Geometry check sheet. Reference: the model listing, model coordinates, mm. A direction names the side the tool comes from. Give positions to 0.01 mm unless a question says otherwise; leave off trailing zeros. Loops run counter-clockwise (first coordinate to the right, second up) from the corner with the lowest first, then second, coordinate; pieces in that order, holes last. Notation, with made-up numbers: (36.25, 70.25) - (95.25, 70.25) arc R19 cw to (95.25, 78.25) - close; hole circle Ø8 at (44, 68.25). An arc over 180 degrees is marked (long way). One line per question, with ' | ' between items. Start each with the question number.
from build123d import *

# Parameters (mm, degrees)
SKETCH1_R           = 1.25
SKETCH1_R_2         = 0.75
SKETCH1_W           = 60
SKETCH1_H           = 20
SKETCH1_W_2         = 5
SKETCH1_H_2         = 1
BOSS_EXTRUDE2_DEPTH = 3
SKETCH4_R           = 0.75
CUT_EXTRUDE3_DEPTH  = 3
SKETCH5_R           = 0.75
CUT_EXTRUDE4_DEPTH  = 3
SKETCH14_R          = 0.75
CUT_EXTRUDE12_DEPTH = 10
BOSS_EXTRUDE4_START = -3
SKETCH15_R          = 0.75
BOSS_EXTRUDE4_DEPTH = 3
SKETCH20_R          = 1.25
CUT_EXTRUDE17_DEPTH = 3
SKETCH23_R          = 0.75
CUT_EXTRUDE21_DEPTH = 10
SKETCH25_W          = 10
SKETCH25_H          = 1
CUT_EXTRUDE23_DEPTH = 3
SKETCH26_R          = 1.25
CUT_EXTRUDE24_DEPTH = 3
SKETCH29_R          = 1.25
CUT_EXTRUDE27_DEPTH = 3
SKETCH33_W          = 5
SKETCH33_H          = 2
CUT_EXTRUDE31_DEPTH = 3
SKETCH34_W          = 5
SKETCH34_H          = 2
CUT_EXTRUDE32_DEPTH = 3
SKETCH35_R          = 1.25
CUT_EXTRUDE33_DEPTH = 3
SKETCH37_R          = 1.25
CUT_EXTRUDE34_DEPTH = 3
SKETCH38_R          = 1.25
CUT_EXTRUDE35_DEPTH = 3
SKETCH41_R          = 0.75
CUT_EXTRUDE38_DEPTH = 3
SKETCH42_W          = 6
SKETCH42_H          = 2
CUT_EXTRUDE40_DEPTH = 3
SKETCH43_W          = 6
SKETCH43_H          = 2
CUT_EXTRUDE41_DEPTH = 3
BOSS_EXTRUDE5_START = -3
SKETCH45_R          = 1.25
BOSS_EXTRUDE5_DEPTH = 3
BOSS_EXTRUDE6_START = -3
SKETCH46_R          = 1.25
BOSS_EXTRUDE6_DEPTH = 3
SKETCH47_R          = 1.25
CUT_EXTRUDE42_DEPTH = 3
SKETCH49_R          = 1.25
CUT_EXTRUDE43_DEPTH = 3
SKETCH51_R          = 1.25
CUT_EXTRUDE44_DEPTH = 3
SKETCH52_R          = 1.25
CUT_EXTRUDE45_DEPTH = 3
SKETCH53_R          = 1.25
CUT_EXTRUDE46_DEPTH = 3
SKETCH54_R          = 1.25
CUT_EXTRUDE47_DEPTH = 3
SKETCH55_W          = 20
SKETCH55_H          = 1
CUT_EXTRUDE48_DEPTH = 10
SKETCH56_R          = 0.75
CUT_EXTRUDE49_DEPTH = 10
SKETCH57_R          = 0.75
CUT_EXTRUDE50_DEPTH = 10
SKETCH59_R          = 1.5
CUT_EXTRUDE51_DEPTH = 10
SKETCH60_R          = 0.75
CUT_EXTRUDE52_DEPTH = 10
SKETCH61_R          = 0.75
CUT_EXTRUDE53_DEPTH = 10
SKETCH65_R          = 1.5
CUT_EXTRUDE55_DEPTH = 10
SKETCH66_R          = 1.5
CUT_EXTRUDE56_DEPTH = 10
SKETCH67_R          = 1.5
CUT_EXTRUDE57_DEPTH = 10
CUT_EXTRUDE58_DEPTH = 10
CUT_EXTRUDE59_DEPTH = 10
BOSS_EXTRUDE7_DEPTH = 3


with BuildPart() as part:
    # Sketch1 → Boss-Extrude2 (new body)
    with BuildSketch(Plane.XY):
        Polygon((58.345821786, 13.119852123), (58.345821786, -56.880147877), (-191.654178214, -56.880147877), (-191.654178214, -26.880147877), (-221.654178214, -6.880147877), (-221.654178214, 33.119852123), (-121.654178214, 33.119852123), (-91.654178214, 13.119852123), align=None)
        with Locations((53.345821786, 7.945541925)):
            Circle(SKETCH1_R, mode=Mode.SUBTRACT)
        with Locations((53.345821786, -52.054458075)):
            Circle(SKETCH1_R, mode=Mode.SUBTRACT)
        with Locations((25.505821786, -18.330147877)):
            Circle(SKETCH1_R_2, mode=Mode.SUBTRACT)
        with Locations((-181.654178214, 13.119852123)):
            Rectangle(SKETCH1_W, SKETCH1_H, mode=Mode.SUBTRACT)
        with Locations((25.845821786, 10.619852123)):
            Rectangle(SKETCH1_W_2, SKETCH1_H_2, mode=Mode.SUBTRACT)
        with Locations((40.845821786, 10.619852123)):
            Rectangle(SKETCH1_W_2, SKETCH1_H_2, mode=Mode.SUBTRACT)
    extrude(amount=BOSS_EXTRUDE2_DEPTH)

    # Sketch4 → Cut-Extrude3 (cut)
    with BuildSketch(Plane.XY.offset(3)):
        with Locations((-12.554178214, -8.780147877)):
            Circle(SKETCH4_R)
    extrude(amount=-CUT_EXTRUDE3_DEPTH, mode=Mode.SUBTRACT)

    # Sketch5 → Cut-Extrude4 (cut)
    with BuildSketch(Plane.XY.offset(3)):
        with Locations((-13.994178214, -15.020147877)):
            Circle(SKETCH5_R)
    extrude(amount=-CUT_EXTRUDE4_DEPTH, mode=Mode.SUBTRACT)

    # Sketch14 → Cut-Extrude12 (cut)
    with BuildSketch(Plane.XY.offset(3)):
        with Locations((25.505821786, -20.330147877)):
            Circle(SKETCH14_R)
        with Locations((25.505821786, -26.730147877)):
            Circle(SKETCH14_R)
    extrude(amount=-CUT_EXTRUDE12_DEPTH, mode=Mode.SUBTRACT)

    # Sketch15 → Boss-Extrude4 (add)
    with BuildSketch(Plane.XY.offset(3).offset(BOSS_EXTRUDE4_START)):
        with Locations((25.505821786, -18.330147877)):
            Circle(SKETCH15_R)
    extrude(amount=BOSS_EXTRUDE4_DEPTH)

    # Sketch20 → Cut-Extrude17 (cut)
    with BuildSketch(Plane.XY.offset(3)):
        with Locations((-16.654178214, 4.119852123)):
            Circle(SKETCH20_R)
    extrude(amount=-CUT_EXTRUDE17_DEPTH, mode=Mode.SUBTRACT)

    # Sketch23 → Cut-Extrude21 (cut)
    with BuildSketch(Plane.XY.offset(3)):
        with Locations((-93.524701832, -7.521447448)):
            Circle(SKETCH23_R)
    extrude(amount=-CUT_EXTRUDE21_DEPTH, mode=Mode.SUBTRACT)

    # Sketch25 → Cut-Extrude23 (cut)
    with BuildSketch(Plane.XY.offset(3)):
        with Locations((33.345821786, 10.619852123)):
            Rectangle(SKETCH25_W, SKETCH25_H)
    extrude(amount=-CUT_EXTRUDE23_DEPTH, mode=Mode.SUBTRACT)

    # Sketch26 → Cut-Extrude24 (cut)
    with BuildSketch(Plane.XY.offset(3)):
        with Locations((-97.444178214, 7.419852123)):
            Circle(SKETCH26_R)
    extrude(amount=-CUT_EXTRUDE24_DEPTH, mode=Mode.SUBTRACT)

    # Sketch29 → Cut-Extrude27 (cut)
    with BuildSketch(Plane.XY.offset(3)):
        with Locations((-176.654178214, -41.880147877)):
            Circle(SKETCH29_R)
    extrude(amount=-CUT_EXTRUDE27_DEPTH, mode=Mode.SUBTRACT)

    # Sketch33 → Cut-Extrude31 (cut)
    with BuildSketch(Plane.XY.offset(3)):
        with Locations((-129.154178214, 30.119852123)):
            Rectangle(SKETCH33_W, SKETCH33_H)
    extrude(amount=-CUT_EXTRUDE31_DEPTH, mode=Mode.SUBTRACT)

    # Sketch34 → Cut-Extrude32 (cut)
    with BuildSketch(Plane.XY.offset(3)):
        with Locations((-144.154178214, 30.119852123)):
            Rectangle(SKETCH34_W, SKETCH34_H)
    extrude(amount=-CUT_EXTRUDE32_DEPTH, mode=Mode.SUBTRACT)

    # Sketch35 → Cut-Extrude33 (cut)
    with BuildSketch(Plane.XY.offset(3)):
        with Locations((-123.654178214, 30.119852123)):
            Circle(SKETCH35_R)
        with Locations((-149.654178214, 30.119852123)):
            Circle(SKETCH35_R)
    extrude(amount=-CUT_EXTRUDE33_DEPTH, mode=Mode.SUBTRACT)

    # Sketch37 → Cut-Extrude34 (cut)
    with BuildSketch(Plane.XY.offset(3)):
        with Locations((-61.654178214, -1.880147877)):
            Circle(SKETCH37_R)
    extrude(amount=-CUT_EXTRUDE34_DEPTH, mode=Mode.SUBTRACT)

    # Sketch38 → Cut-Extrude35 (cut)
    with BuildSketch(Plane.XY.offset(3)):
        with Locations((-87.444178214, -25.580147877)):
            Circle(SKETCH38_R)
    extrude(amount=-CUT_EXTRUDE35_DEPTH, mode=Mode.SUBTRACT)

    # Sketch41 → Cut-Extrude38 (cut)
    with BuildSketch(Plane.XY.offset(3)):
        with Locations((-112.306137726, -10.395062897)):
            Circle(SKETCH41_R)
    extrude(amount=-CUT_EXTRUDE38_DEPTH, mode=Mode.SUBTRACT)

    # Sketch42 → Cut-Extrude40 (cut)
    with BuildSketch(Plane.XY.offset(3)):
        with Locations((-105.524701832, -12.521447448)):
            Rectangle(SKETCH42_W, SKETCH42_H)
    extrude(amount=-CUT_EXTRUDE40_DEPTH, mode=Mode.SUBTRACT)

    # Sketch43 → Cut-Extrude41 (cut)
    with BuildSketch(Plane.XY.offset(3)):
        with Locations((-105.524701832, 14.478552552)):
            Rectangle(SKETCH43_W, SKETCH43_H)
    extrude(amount=-CUT_EXTRUDE41_DEPTH, mode=Mode.SUBTRACT)

    # Sketch45 → Boss-Extrude5 (add)
    with BuildSketch(Plane.XY.offset(3).offset(BOSS_EXTRUDE5_START)):
        with Locations((53.345821786, -52.054458075)):
            Circle(SKETCH45_R)
    extrude(amount=BOSS_EXTRUDE5_DEPTH)

    # Sketch46 → Boss-Extrude6 (add)
    with BuildSketch(Plane.XY.offset(3).offset(BOSS_EXTRUDE6_START)):
        with Locations((53.345821786, 7.945541925)):
            Circle(SKETCH46_R)
    extrude(amount=BOSS_EXTRUDE6_DEPTH)

    # Sketch47 → Cut-Extrude42 (cut)
    with BuildSketch(Plane.XY.offset(3)):
        with Locations((53.345821786, 8.119852123)):
            Circle(SKETCH47_R)
    extrude(amount=-CUT_EXTRUDE42_DEPTH, mode=Mode.SUBTRACT)

    # Sketch49 → Cut-Extrude43 (cut)
    with BuildSketch(Plane.XY.offset(3)):
        with Locations((53.345821786, -10.880147877)):
            Circle(SKETCH49_R)
    extrude(amount=-CUT_EXTRUDE43_DEPTH, mode=Mode.SUBTRACT)

    # Sketch51 → Cut-Extrude44 (cut)
    with BuildSketch(Plane.XY.offset(3)):
        with Locations((53.345821786, -36.880147877)):
            Circle(SKETCH51_R)
    extrude(amount=-CUT_EXTRUDE44_DEPTH, mode=Mode.SUBTRACT)

    # Sketch52 → Cut-Extrude45 (cut)
    with BuildSketch(Plane.XY.offset(3)):
        with Locations((53.345821786, -51.880147877)):
            Circle(SKETCH52_R)
    extrude(amount=-CUT_EXTRUDE45_DEPTH, mode=Mode.SUBTRACT)

    # Sketch53 → Cut-Extrude46 (cut)
    with BuildSketch(Plane.XY.offset(3)):
        with Locations((-6.654178214, -51.880147877)):
            Circle(SKETCH53_R)
    extrude(amount=-CUT_EXTRUDE46_DEPTH, mode=Mode.SUBTRACT)

    # Sketch54 → Cut-Extrude47 (cut)
    with BuildSketch(Plane.XY.offset(3)):
        with Locations((-61.654178214, -51.880147877)):
            Circle(SKETCH54_R)
    extrude(amount=-CUT_EXTRUDE47_DEPTH, mode=Mode.SUBTRACT)

    # Sketch55 → Cut-Extrude48 (cut)
    with BuildSketch(Plane.XY.offset(3)):
        with Locations((33.345821786, 9.619852123)):
            Rectangle(SKETCH55_W, SKETCH55_H)
    extrude(amount=-CUT_EXTRUDE48_DEPTH, mode=Mode.SUBTRACT)

    # Sketch56 → Cut-Extrude49 (cut)
    with BuildSketch(Plane.XY.offset(3)):
        with Locations((-61.804178214, -20.030147877)):
            Circle(SKETCH56_R)
    extrude(amount=-CUT_EXTRUDE49_DEPTH, mode=Mode.SUBTRACT)

    # Sketch57 → Cut-Extrude50 (cut)
    with BuildSketch(Plane.XY.offset(3)):
        with Locations((-79.304178214, -20.030147877)):
            Circle(SKETCH57_R)
    extrude(amount=-CUT_EXTRUDE50_DEPTH, mode=Mode.SUBTRACT)

    # Sketch59 → Cut-Extrude51 (cut)
    with BuildSketch(Plane.XY.offset(3)):
        with Locations((-87.444178214, -42.580147877)):
            Circle(SKETCH59_R)
    extrude(amount=-CUT_EXTRUDE51_DEPTH, mode=Mode.SUBTRACT)

    # Sketch60 → Cut-Extrude52 (cut)
    with BuildSketch(Plane.XY.offset(3)):
        with Locations((-18.804178214, -26.030147877)):
            Circle(SKETCH60_R)
    extrude(amount=-CUT_EXTRUDE52_DEPTH, mode=Mode.SUBTRACT)

    # Sketch61 → Cut-Extrude53 (cut)
    with BuildSketch(Plane.XY.offset(3)):
        with Locations((-36.304178214, -26.030147877)):
            Circle(SKETCH61_R)
    extrude(amount=-CUT_EXTRUDE53_DEPTH, mode=Mode.SUBTRACT)

    # Sketch65 → Cut-Extrude55 (cut)
    with BuildSketch(Plane.XY.offset(3)):
        with Locations((1.345821786, 3.119852123)):
            Circle(SKETCH65_R)
    extrude(amount=-CUT_EXTRUDE55_DEPTH, mode=Mode.SUBTRACT)

    # Sketch66 → Cut-Extrude56 (cut)
    with BuildSketch(Plane.XY.offset(3)):
        with Locations((-107.444178214, -29.580147877)):
            Circle(SKETCH66_R)
    extrude(amount=-CUT_EXTRUDE56_DEPTH, mode=Mode.SUBTRACT)

    # Sketch67 → Cut-Extrude57 (cut)
    with BuildSketch(Plane.XY.offset(3)):
        with Locations((-127.444178214, -20.580147877)):
            Circle(SKETCH67_R)
    extrude(amount=-CUT_EXTRUDE57_DEPTH, mode=Mode.SUBTRACT)

    # Sketch68 → Cut-Extrude58 (cut)
    with BuildSketch(Plane.XY.offset(3)):
        with BuildLine():
            Line((-221.654178214, 33.119852123), (-216.654178214, 33.119852123))
            ThreePointArc((-216.654178214, 33.119852123), (-220.18971212, 31.655386029), (-221.654178214, 28.119852123))
            Line((-221.654178214, 28.119852123), (-221.654178214, 33.119852123))
        make_face()
    extrude(amount=-CUT_EXTRUDE58_DEPTH, mode=Mode.SUBTRACT)

    # Sketch69 → Cut-Extrude59 (cut)
    with BuildSketch(Plane.XY.offset(3)):
        with BuildLine():
            Line((-191.654178214, -56.880147877), (-191.654178214, -51.880147877))
            ThreePointArc((-191.654178214, -51.880147877), (-190.18971212, -55.415681783), (-186.654178214, -56.880147877))
            Line((-186.654178214, -56.880147877), (-191.654178214, -56.880147877))
        make_face()
    extrude(amount=-CUT_EXTRUDE59_DEPTH, mode=Mode.SUBTRACT)

    # Sketch72 → Boss-Extrude7 (add)
    with BuildSketch(Plane.XY.offset(3)):
        with BuildLine():
            Line((-211.654178214, 23.119852123), (-211.654178214, 18.119852123))
            ThreePointArc((-211.654178214, 18.119852123), (-210.18971212, 21.655386029), (-206.654178214, 23.119852123))
            Line((-206.654178214, 23.119852123), (-211.654178214, 23.119852123))
        make_face()
        with BuildLine():
            Line((-211.654178214, 3.119852123), (-211.654178214, 8.119852123))
            ThreePointArc((-211.654178214, 8.119852123), (-210.18971212, 4.584318217), (-206.654178214, 3.119852123))
            Line((-206.654178214, 3.119852123), (-211.654178214, 3.119852123))
        make_face()
        with BuildLine():
            Line((-151.654178214, 23.119852123), (-156.654178214, 23.119852123))
            ThreePointArc((-156.654178214, 23.119852123), (-153.118644308, 21.655386029), (-151.654178214, 18.119852123))
            Line((-151.654178214, 18.119852123), (-151.654178214, 23.119852123))
        make_face()
        with BuildLine():
            Line((-151.654178214, 3.119852123), (-156.654178214, 3.119852123))
            ThreePointArc((-156.654178214, 3.119852123), (-153.118644308, 4.584318217), (-151.654178214, 8.119852123))
            Line((-151.654178214, 8.119852123), (-151.654178214, 3.119852123))
        make_face()
    extrude(amount=-BOSS_EXTRUDE7_DEPTH)


solid = part.part
(1) Section check C-C, the plane z = 1.7. Count the separate pieces of the cut face and the enclosed holes in it, and give its area (3 significant figures).
(2) Material ranges on line 1 (Y direction, x = -174.5, z = 2.4); line 2 (X direction, y = 8, z = 2.4); line 3 (X direction, y = 29, z = 2.05), recorded low to high.
(3) Section check B-B, the plane x = -204. Record the boundary of the cut face in (y, z).
(4) Tool access check on faces 5 (the face through (-210.228, 4.623, 1.521)), 6 (the face through (-190.228, -55.377, 1.521)). Record the directions out of +Z, -Z, +X, -X, +Y, -Y that give a thin tool (end or side, any length) a straight path to the whole face; none if there is none.
(5) Section check A-A, the plane x = 30. Record the boundary of the cut face in (y, z).
(6) Mould release check, pull along X, two halves, no side actions. Record for faces 1 (the face through (-206.444, -17.02, 1.479)), 2 (the face through (-153.158, 21.694, 1.521)), 3 (the face through (-84, -21, 3)), 4 (the face through (-153.158, 4.546, 1.521)): pulls with the +X half, pulls with the -X half, needs draft (parallel to the pull), parting line crosses it, or undercut.
(7) Depth check by flat-ended pin: pin 1 Ø1.5 at (x, z) = (-104.5, 1) entering from +Y. Enter the tip coordinate at first touch or a pass-through.
Numbers:
1) separate pieces: 1 | enclosed holes: 33 | area: 19,300 mm^2
2) line 1: -56.88 to 3.12, 23.12 to 33.12 | line 2: -221.65 to -211.65, -151.66 to -98.55, -96.34 to 52.1, 54.59 to 58.35 | line 3: -221.58 to -150.21, -149.1 to -124.21, -123.1 to -115.47
3) outline: (-18.65, 0) - (3.12, 0) - (3.12, 3) - (-18.65, 3) - close; (23.12, 0) - (33.12, 0) - (33.12, 3) - (23.12, 3) - close
4) face 5: +Z, -Z | face 6: +Z, -Z, -X, -Y
5) outline: (-56.88, 0) - (9.12, 0) - (9.12, 3) - (-56.88, 3) - close; (11.12, 0) - (13.12, 0) - (13.12, 3) - (11.12, 3) - close
6) face 1: pulls with the -X half | face 2: undercut | face 3: needs draft | face 4: undercut
7) pin 1: y = 22.18
